Input: part model. Units: mm. Frame: model coordinates. Coordinates: 2 decimals unless noted, no trailing zeros. Write each loop counter-clockwise with the first axis right and the second up, starting at its lowest first coordinate (ties: lowest second). Pieces come first, ordered by that corner, then holes. Notation, with made-up numbers: M 71,4.25 L 129,4.25 A31 ccw 129,42.25 Z; hole C 70,38.5 d7. An arc over 180 degrees is marked long. Use one line per item in the form item = value.
from build123d import *

# Parameters (mm, degrees)
SKIZZE1_R                       = 12.5
SKIZZE1_R_2                     = 5
AUFSATZ_LINEAR_AUSTRAGEN1_DEPTH = 25
SKIZZE2_R                       = 1
SCHNITT_LINEAR_AUSTRAGEN1_DEPTH = 25


with BuildPart() as part:
    # Skizze1 → Aufsatz-Linear austragen1 (new body)
    with BuildSketch(Plane.XY):
        Circle(SKIZZE1_R)
        Circle(SKIZZE1_R_2, mode=Mode.SUBTRACT)
    extrude(amount=AUFSATZ_LINEAR_AUSTRAGEN1_DEPTH)

    # Skizze2 → Schnitt-Linear austragen1 (cut)
    with BuildSketch(Plane.XY.offset(25)):
        with Locations((0, 8.75)):
            Circle(SKIZZE2_R)
        with Locations((6.187184335, 6.187184335)):
            Circle(SKIZZE2_R)
        with Locations((8.75, 0)):
            Circle(SKIZZE2_R)
        with Locations((6.187184335, -6.187184335)):
            Circle(SKIZZE2_R)
        with Locations((0, -8.75)):
            Circle(SKIZZE2_R)
        with Locations((-6.187184335, -6.187184335)):
            Circle(SKIZZE2_R)
        with Locations((-8.75, 0)):
            Circle(SKIZZE2_R)
        with Locations((-6.187184335, 6.187184335)):
            Circle(SKIZZE2_R)
    extrude(amount=-SCHNITT_LINEAR_AUSTRAGEN1_DEPTH, mode=Mode.SUBTRACT)


solid = part.part
(1) Section query C-C on z = 21. State how many separate pieces and enclosed holes the cut face has, plus the area to 3 significant figures.
Computed:
separate_pieces = 1
enclosed_holes = 9
area = 387 mm^2
(2) First-contact query: pin 1 Ø12 at (x, z) = (-4, 17) entering from +Y; pin 2 Ø6 at (x, z) = (4.5, 14.5) entering from +Y; pin 3 Ø1 at (x, z) = (5, 4) entering from -Y; pin 4 Ø4 at (y, z) = (4, 21.5) entering from +X. Flat tips, straight axial feed; report the tip coordinate or a pass-through.
Computed:
pin_1 = 12.5
pin_2 = 12.41
pin_3 = -11.66
pin_4 = 12.34
(3) Section query B-B on x = 6. Return the cut outline in (y, z).
Computed:
outline = M -10.97,0 L -7.17,0 L -7.17,25 L -10.97,25 Z; M -5.2,0 L 5.2,0 L 5.2,25 L -5.2,25 Z; M 7.17,0 L 10.97,0 L 10.97,25 L 7.17,25 Z
(4) Line query: probe 1 along Y at (x, z) = (0, 9.25); probe 2 along X at (y, z) = (-6.75, 17); probe 3 along X at (y, z) = (7, 22). Output: solid intervals per line, ascending.
Computed:
probe_1 = -12.5 to -9.75, -7.75 to -5, 5 to 7.75, 9.75 to 12.5
probe_2 = -10.52 to -7.01, -5.36 to 5.36, 7.01 to 10.52
probe_3 = -10.36 to -6.77, -5.6 to 5.6, 6.77 to 10.36
(5) Pull-direction query (Y, two-part tool) for faces 1 (the cylindrical face through (11.923, 3.755, 12.325)), 2 (the cylindrical face through (-6.4, 5.21, 12.68)), 3 (the flat face through (-0.2, -5.4, 25)); classes: pulls with the +Y half, pulls with the -Y half, needs draft (parallel to the pull), parting line crosses it, or undercut.
Computed:
face_1 = parting line crosses it
face_2 = undercut
face_3 = needs draft
(6) Section query A-A on y = 6.75. Return the cut outline in (x, z).
Computed:
outline = M -10.52,0 L -7.01,0 L -7.01,25 L -10.52,25 Z; M -5.36,0 L 5.36,0 L 5.36,25 L -5.36,25 Z; M 7.01,0 L 10.52,0 L 10.52,25 L 7.01,25 Z
(7) Section query D-D on y = 0. Return the cut outline in (x, z).
Computed:
outline = M -12.5,0 L -9.75,0 L -9.75,25 L -12.5,25 Z; M -7.75,0 L -5,0 L -5,25 L -7.75,25 Z; M 5,0 L 7.75,0 L 7.75,25 L 5,25 Z; M 9.75,0 L 12.5,0 L 12.5,25 L 9.75,25 Z
